Here's the drawing with two shaded views (mm, measured from the low corner). I have some questions. Coordinates: 2 decimals unless noted, no trailing zeros. Loops run counter-clockwise (first coordinate to the right, second up) from the corner with the lowest first, then second, coordinate; pieces in that order, holes last. Notation, with made-up numbers: M 73.5,38 L 111.5,38 A17 ccw 111.5,67 Z; hole C 12,37.5 d4. An arc over 180 degrees is marked long. Return JSON: item names as keys, results as strings. Group by question number.
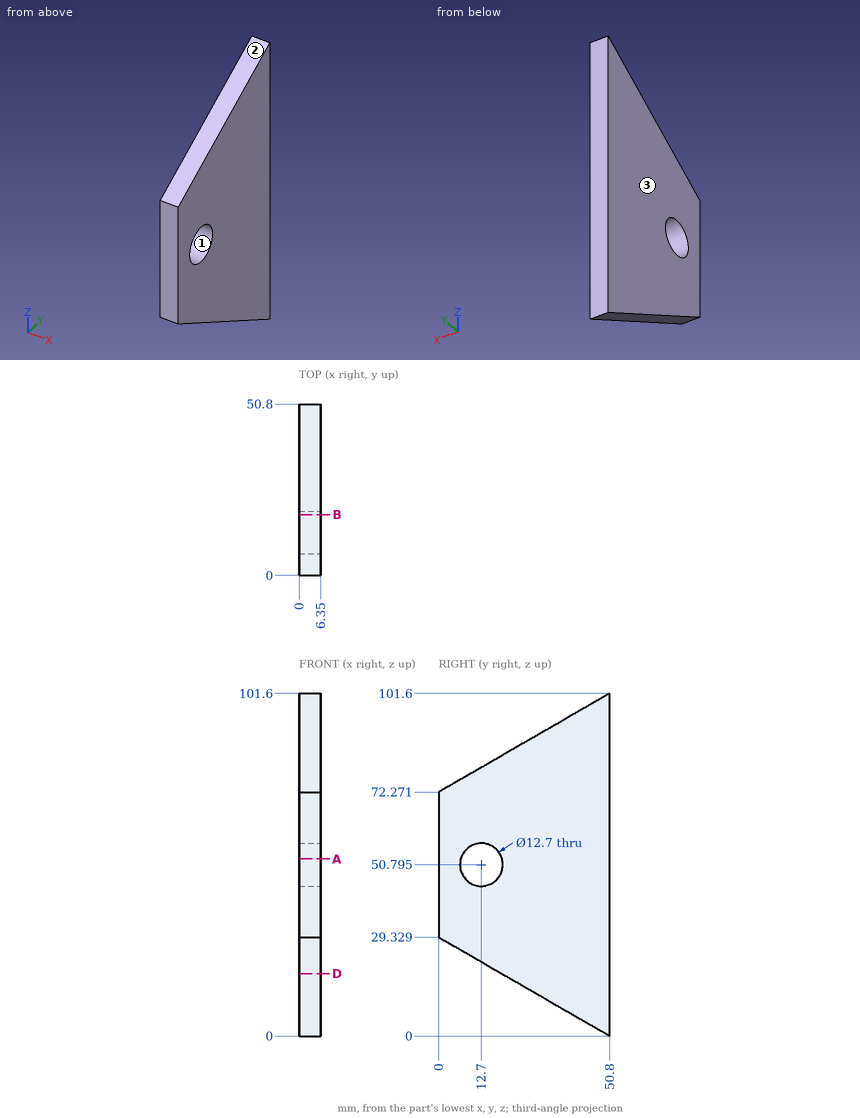
1) Suppose I cut it at A-A, the plane z = 52.5. List the corners of the cut face in (x, y) for me.
2) If I drill on line 1 (Z direction, x = 2.75, y = 12.7) (1 decimal); line 2 (Z direction, x = 4, y = 13) (1 decimal); line 3 (Z direction, x = 4.5, y = 37.5), over which ranges is the centre line in solid material (lowest first)? Write a range as from..to.
3) If we mould it in two halves opening along Z, with no side actions, what happens to the marked faces 1, 2 and 3? For each: +Z half, -Z half, draft (parallel to the pull), parting line (faces both ways), or undercut.
4) Suppose I cut it at D-D, the plane z = 18.5. List the corners of the cut face in (x, y) for me.
5) Suppose I cut it at B-B, the plane y = 18. List the corners of the cut face in (x, z) for me.
Returned:
{
 "1": {"outline": "M 0,0 L 6.35,0 L 6.35,6.58 L 0,6.58 Z; M 0,18.82 L 6.35,18.82 L 6.35,50.8 L 0,50.8 Z"},
 "2": {"line 1": "z = 22..44.4, 57.1..79.6", "line 2": "z = 21.8..44.5, 57.1..79.8", "line 3": "z = 7.68..93.92"},
 "3": {"face 1": "undercut", "face 2": "+Z half", "face 3": "draft"},
 "4": {"outline": "M 0,18.76 L 6.35,18.76 L 6.35,50.8 L 0,50.8 Z"},
 "5": {"outline": "M 0,18.94 L 6.35,18.94 L 6.35,47.3 L 0,47.3 Z; M 0,54.29 L 6.35,54.29 L 6.35,82.66 L 0,82.66 Z"}
}
